from build123d import *

# Parameters (mm, degrees)
ESQUISSE1_W             = 85
ESQUISSE1_H             = 70
BOSS_EXTRU_1_DEPTH      = 2.5
ESQUISSE2_W             = 85
ESQUISSE2_H             = 70
ESQUISSE2_W_2           = 80
ESQUISSE2_H_2           = 65
BOSS_EXTRU_2_DEPTH      = 17.1
ESQUISSE3_R             = 2.75
ESQUISSE3_R_2           = 1.5
BOSS_EXTRU_3_DEPTH      = 4
CHANFREIN1_SIZE         = 4.5
CHANFREIN2_SIZE         = 4
ESQUISSE4_R             = 5
ENL_V_MAT_EXTRU_1_DEPTH = 10


with BuildPart() as part:
    # Esquisse1 → Boss.-Extru.1 (new body)
    with BuildSketch(Plane.XY):
        with Locations((42.5, 35)):
            Rectangle(ESQUISSE1_W, ESQUISSE1_H)
    extrude(amount=BOSS_EXTRU_1_DEPTH)

    # Esquisse2 → Boss.-Extru.2 (add)
    with BuildSketch(Plane.XY.offset(2.5)):
        with Locations((42.5, 35)):
            Rectangle(ESQUISSE2_W, ESQUISSE2_H)
        with Locations((42.5, 35)):
            Rectangle(ESQUISSE2_W_2, ESQUISSE2_H_2, mode=Mode.SUBTRACT)
    extrude(amount=BOSS_EXTRU_2_DEPTH)

    # Esquisse3 → Boss.-Extru.3 (add)
    # profile 1 of 4: a face of its own
    with BuildSketch(Plane.XY.offset(2.5)):
        with Locations(Location((8.21, 61.19, 0), (0, 0, 180))):
            Circle(ESQUISSE3_R)
        with Locations((8.21, 61.19)):
            Circle(ESQUISSE3_R_2, mode=Mode.SUBTRACT)
    # profile 2 of 4: a face of its own
    with BuildSketch(Plane.XY.offset(2.5)):
        with Locations(Location((76.79, 61.19, 0), (0, 0, 180))):
            Circle(ESQUISSE3_R)
        with Locations((76.79, 61.19)):
            Circle(ESQUISSE3_R_2, mode=Mode.SUBTRACT)
    # profile 3 of 4: a face of its own
    with BuildSketch(Plane.XY.offset(2.5)):
        with Locations(Location((76.79, 10.39, 0), (0, 0, 180))):
            Circle(ESQUISSE3_R)
        with Locations((76.79, 10.39)):
            Circle(ESQUISSE3_R_2, mode=Mode.SUBTRACT)
    # profile 4 of 4: a face of its own
    with BuildSketch(Plane.XY.offset(2.5)):
        with Locations(Location((8.21, 10.39, 0), (0, 0, 180))):
            Circle(ESQUISSE3_R)
        with Locations((8.21, 10.39)):
            Circle(ESQUISSE3_R_2, mode=Mode.SUBTRACT)
    extrude(amount=BOSS_EXTRU_3_DEPTH)

    # Chanfrein1
    chanfrein1_edges = [part.edges().sort_by_distance(p)[0] for p in [
        (2.5, 67.5, 11.05),
        (2.5, 2.5, 11.05),
        (82.5, 2.5, 11.05),
        (82.5, 67.5, 11.05),
        (0, 70, 9.8),
        (85, 70, 9.8),
        (85, 0, 9.8),
        (0, 0, 9.8),
    ]]
    chamfer(chanfrein1_edges, length=CHANFREIN1_SIZE)

    # Chanfrein2
    # the kernel refuses this chamfer: 4 mm, written as the material it adds along each edge
    with BuildSketch(Plane(origin=(8.21, 10.39, 2.5), x_dir=(-1, 0, 0), z_dir=(0, 1, 0))) as chanfrein2_piece_1_section:
        Polygon((2.75 + CHANFREIN2_SIZE, 0), (2.75, CHANFREIN2_SIZE), (2.75, 0), align=None)
    chanfrein2_piece_1 = revolve(axis=Axis((8.21, 10.39, 2.5), (0, 0, 1)), mode=Mode.PRIVATE)
    chanfrein2_piece_1 = split(chanfrein2_piece_1, bisect_by=Plane(origin=(12.973571243, 10.39, 6.5), z_dir=(0, 0, -1)), keep=Keep.TOP, mode=Mode.PRIVATE)
    add(chanfrein2_piece_1)
    with BuildSketch(Plane(origin=(76.79, 10.39, 2.5), x_dir=(-1, 0, 0), z_dir=(0, 1, 0))) as chanfrein2_piece_2_section:
        Polygon((2.75 + CHANFREIN2_SIZE, 0), (2.75, CHANFREIN2_SIZE), (2.75, 0), align=None)
    chanfrein2_piece_2 = revolve(axis=Axis((76.79, 10.39, 2.5), (0, 0, 1)), mode=Mode.PRIVATE)
    chanfrein2_piece_2 = split(chanfrein2_piece_2, bisect_by=Plane(origin=(81.553571243, 10.39, 6.5), z_dir=(0, 0, -1)), keep=Keep.TOP, mode=Mode.PRIVATE)
    add(chanfrein2_piece_2)
    with BuildSketch(Plane(origin=(76.79, 61.19, 2.5), x_dir=(-1, 0, 0), z_dir=(0, 1, 0))) as chanfrein2_piece_3_section:
        Polygon((2.75 + CHANFREIN2_SIZE, 0), (2.75, CHANFREIN2_SIZE), (2.75, 0), align=None)
    chanfrein2_piece_3 = revolve(axis=Axis((76.79, 61.19, 2.5), (0, 0, 1)), mode=Mode.PRIVATE)
    chanfrein2_piece_3 = split(chanfrein2_piece_3, bisect_by=Plane(origin=(81.553571243, 61.19, 6.5), z_dir=(0, 0, -1)), keep=Keep.TOP, mode=Mode.PRIVATE)
    add(chanfrein2_piece_3)
    with BuildSketch(Plane(origin=(8.21, 61.19, 2.5), x_dir=(-1, 0, 0), z_dir=(0, 1, 0))) as chanfrein2_piece_4_section:
        Polygon((2.75 + CHANFREIN2_SIZE, 0), (2.75, CHANFREIN2_SIZE), (2.75, 0), align=None)
    chanfrein2_piece_4 = revolve(axis=Axis((8.21, 61.19, 2.5), (0, 0, 1)), mode=Mode.PRIVATE)
    chanfrein2_piece_4 = split(chanfrein2_piece_4, bisect_by=Plane(origin=(12.973571243, 61.19, 6.5), z_dir=(0, 0, -1)), keep=Keep.TOP, mode=Mode.PRIVATE)
    add(chanfrein2_piece_4)

    # Esquisse4 → Enlèv. mat.-Extru.1 (cut)
    with BuildSketch(Plane(origin=(0, 70, 0), x_dir=(1, 0, 0), z_dir=(0, 1, 0))):
        with Locations(Location((42.5, -9.8, 0), (0, 0, 270))):
            Circle(ESQUISSE4_R)
    extrude(amount=-ENL_V_MAT_EXTRU_1_DEPTH, mode=Mode.SUBTRACT)


solid = part.part
Geometry check sheet. Reference: the model listing, model coordinates, mm. A direction names the side the tool comes from. Give positions to 0.01 mm unless a question says otherwise; leave off trailing zeros. Order: outer loops, then holes, each group sorted by start corner. A loop starts at its lowest first (then second) coordinate and runs counter-clockwise, first axis right, second up.
1. Sectioned sample at D-D (x = 76.79). Record the boundary of the cut face in (y, z), then the cut area to 3 significant figures.
Completed:
outline: (0, 0) - (70, 0) - (70, 19.6) - (67.5, 19.6) - (67.5, 2.94) - (63.94, 6.5) - (62.69, 6.5) - (62.69, 2.5) - (59.69, 2.5) - (59.69, 6.5) - (58.44, 6.5) - (54.44, 2.5) - (17.14, 2.5) - (13.14, 6.5) - (11.89, 6.5) - (11.89, 2.5) - (8.89, 2.5) - (8.89, 6.5) - (7.64, 6.5) - (3.64, 2.5) - (2.5, 2.5) - (2.5, 19.6) - (0, 19.6) - close
area: 312 mm2
2. Access from +Z, -Z, +X, -X, +Y, -Y to the whole of each face (thin tool, end or side, straight path). Record for faces 1 (the face through (2.5, 35, 11)), 2 (the face through (47.457, 68.768, 9.149)), 3 (the face through (2.3, 2.2, 9.7)).
Completed:
face 1: +Z
face 2: +Y
face 3: +Z, -Z, -X, -Y
3. Draft check along X on faces 4 (the face through (0, 35, 10)), 5 (the face through (82.8, 2.3, 9.7)), 6 (the face through (76, 12, 6.5)). Enter one of: pulls with the +X half, pulls with the -X half, needs draft (parallel to the pull), parting line crosses it, or undercut.
Completed:
face 4: pulls with the -X half
face 5: pulls with the +X half
face 6: undercut
4. Sectioned sample at B-B (y = 10.39). Record the boundary of the cut face in (x, z), then the cut area to 3 significant figures.
Completed:
outline: (0, 0) - (85, 0) - (85, 19.6) - (82.5, 19.6) - (82.5, 3.54) - (79.54, 6.5) - (78.29, 6.5) - (78.29, 2.5) - (75.29, 2.5) - (75.29, 6.5) - (74.04, 6.5) - (70.04, 2.5) - (14.96, 2.5) - (10.96, 6.5) - (9.71, 6.5) - (9.71, 2.5) - (6.71, 2.5) - (6.71, 6.5) - (5.46, 6.5) - (2.5, 3.54) - (2.5, 19.6) - (0, 19.6) - close
area: 349 mm2
5. Depth check by flat-ended pin: pin 1 (6 mm diameter, centred on x = 8, y = 60.5, fed in from +Z). Enter the tip coordinate at first touch or a pass-through.
Completed:
pin 1: stops at z = 6.5
6. Sectioned sample at A-A (x = 42.5). Record the boundary of the cut face in (y, z).
Completed:
outline: (0, 0) - (70, 0) - (70, 4.8) - (67.5, 4.8) - (67.5, 2.5) - (2.5, 2.5) - (2.5, 19.6) - (0, 19.6) - close; (67.5, 14.8) - (70, 14.8) - (70, 19.6) - (67.5, 19.6) - close
7. Scan lines: line 1 (X direction, y = 15.5, z = 12.75); line 2 (Y direction, x = 44, z = 4.75); line 3 (Y direction, x = 8.21, z = 5.25). Record each from-to range of solid material in increasing order.
Completed:
line 1: x = 0 to 2.5, 82.5 to 85
line 2: y = 0 to 2.5, 67.5 to 70
line 3: y = 0 to 2.5, 6.39 to 8.89, 11.89 to 14.39, 57.19 to 59.69, 62.69 to 65.19, 67.5 to 70
8. Sectioned sample at C-C (z = 9.8). Record the boundary of the cut face in (x, y).
Completed:
outline: (0, 4.5) - (4.5, 0) - (80.5, 0) - (85, 4.5) - (85, 65.5) - (80.5, 70) - (47.5, 70) - (47.5, 67.5) - (78, 67.5) - (82.5, 63) - (82.5, 7) - (78, 2.5) - (7, 2.5) - (2.5, 7) - (2.5, 63) - (7, 67.5) - (37.5, 67.5) - (37.5, 70) - (4.5, 70) - (0, 65.5) - close
